For this review, take the finished solid that the model builds, in its own axes (mm). Face numbers are marked on the shaded views. A direction names the side the tool comes from. Coordinates: 2 decimals unless noted, no trailing zeros. Loops run counter-clockwise (first coordinate to the right, second up) from the corner with the lowest first, then second, coordinate; pieces in that order, holes last. Notation, with made-up numbers: M 43,-16.75 L 63,-16.75 A25 ccw 63,6.25 Z; hole C 54,1.25 d2. An arc over 180 degrees is marked long. Answer as a JSON object with one key per item and string values. Group by question number.
Item 1: Mouldability with a two-part tool opening along X and no side actions: class the marked faces 4, 5 and 6 as +X half, -X half, draft (parallel to the pull), parting line (faces both ways), or undercut.
Item 2: Add section A-A (y = 80). State the section outline as (x, z) points.
Item 3: Add section B-B (z = -171). State the section outline as (x, y) points, then the cut area to 3 significant figures.
Item 4: Add section C-C (x = 119). State the section outline as (y, z) points.
Item 5: Wall thickness on L1, parallel to Z at x = 210.5, y = 64.5; L2, parallel to X at y = 118.5, z = -390; L3, parallel to X at y = 9, z = -358: over which ranges is each line inside the solid? List them lowest first. Write a range as from..to.
Item 6: Insertion check: pin 1 (1 mm diameter, centred on y = 116, z = -232, fed in from +X); pin 2 (5 mm diameter, centred on x = 156, z = -265, fed in from +Y); pin 3 (8 mm diameter, centred on y = 132, z = -338.5, fed in from -X). Each pin has a flat end and moves straight along its axis. Give the tip position at first contact, or say it passes through.
Item 7: Tool access review of the marked faces 1, 2 and 3: name each direction out of +Z, -Z, +X, -X, +Y, -Y from which nothing blocks a thin tool from reaching the whole face with its end or side.
Autodesk Inventor part; units mm, degrees
ref_plane "YZ Plane" through (0, 0, 0) normal (1, 0, 0) x (0, 1, 0)
ref_plane "XZ Plane" through (0, 0, 0) normal (0, 1, 0) x (-1, 0, 0)
ref_plane "XY Plane" through (0, 0, 0) normal (0, 0, 1) x (1, 0, 0)
sketch "Sketch5" plane through (0, 0, 0) normal (0, 0, 1) x (1, 0, 0)
  line L0 (0, 0) -> (370, 0)
  line L1 (370, 0) -> (370, 150)
  line L2 (370, 150) -> (0, 150)
  line L3 (0, 150) -> (0, 0)
  dimension "d15" = 370
  dimension "d16" = 150
extrude "Extrusion5" add sketch "Sketch5" along normal blind 18
sketch "Sketch6" plane through (0, 0, 0) normal (0, 0, -1) x (-1, 0, 0)
  line L0 (-362.3, 140) -> (-344.3, 140)
  line L1 (-344.3, 140) -> (-344.3, 5)
  line L2 (-344.3, 5) -> (-362.3, 5)
  line L3 (-362.3, 5) -> (-362.3, 140)
  line L4 (-370, 0) -> (-370, 150)
  line L5 (0, 0) -> (-370, 0)
  line L6 (-25.7, 140) -> (-7.7, 140)
  line L7 (-7.7, 140) -> (-7.7, 5)
  line L8 (-7.7, 5) -> (-25.7, 5)
  line L9 (-25.7, 5) -> (-25.7, 140)
  line L10 (0, 150) -> (0, 0)
  dimension "d19" = 18
  dimension "d20" = 135
  dimension "d21" = 7.7
  dimension "d22" = 5
  dimension "d23" = 18
  dimension "d24" = 7.7
  dimension "d25" = 5
extrude "Extrusion6" add sketch "Sketch6" along normal blind 550
sketch "Sketch7" plane through (0, 0, -550) normal (0, 0, -1) x (-1, 0, 0)
  line L0 (-344.3, 140) -> (-344.3, 5)
  line L1 (-25.7, 5) -> (-25.7, 140)
  line L2 (-344.3, 140) -> (-25.7, 140)
  line L3 (-25.7, 140) -> (-25.7, 5)
  line L4 (-25.7, 5) -> (-344.3, 5)
  line L5 (-344.3, 5) -> (-344.3, 140)
  point P0 (0, 0)
extrude "Extrusion7" add sketch "Sketch7" against normal blind 18
sketch "Sketch8" plane through (7.7, 5, -550) normal (0, -1, 0) x (1, 0, 0)
  line L0 (354.6, 550) -> (336.6, 550)
  line L1 (354.6, 550) -> (354.6, 0)
  line L2 (0, 0) -> (354.6, 0)
  line L3 (0, 550) -> (0, 0)
  line L4 (18, 550) -> (0, 550)
  line L5 (18, 550) -> (18, 18)
  line L6 (336.6, 18) -> (18, 18)
  line L7 (336.6, 550) -> (336.6, 18)
  line L8 (362.3, 550) -> (-7.7, 550)
extrude "Extrusion8" add sketch "Sketch8" against normal blind 9 contours L7 L6 L5 L8
equation "\"d16\" = Cajon02Altura"
equation "\"d24\" = d21"
equation "\"d25\" = d22"
properties part number "FrenteGrande" material "Wood (Birch)"
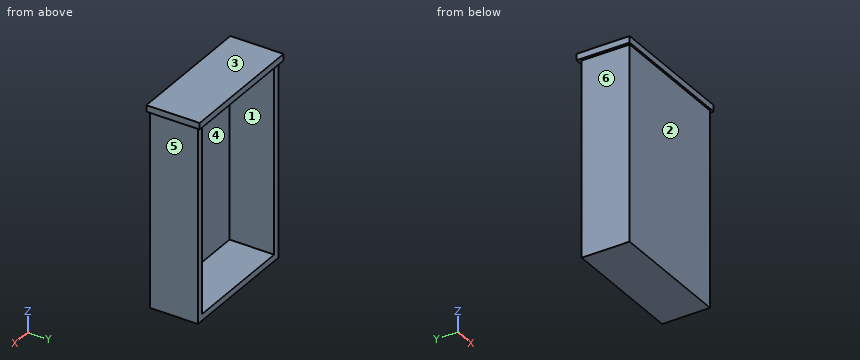
From the geometry:
{
 "1": {"face 4": "undercut", "face 5": "+X half", "face 6": "-X half"},
 "2": {"outline": "M 0,0 L 7.7,0 L 7.7,-550 L 362.3,-550 L 362.3,0 L 370,0 L 370,18 L 0,18 Z; hole M 25.7,-532 L 344.3,-532 L 344.3,0 L 25.7,0 Z"},
 "3": {"outline": "M 7.7,5 L 362.3,5 L 362.3,140 L 344.3,140 L 344.3,14 L 25.7,14 L 25.7,140 L 7.7,140 Z", "area": "7,730 mm²"},
 "4": {"outline": "M 0,0 L 5,0 L 5,-550 L 140,-550 L 140,-532 L 14,-532 L 14,0 L 150,0 L 150,18 L 0,18 Z"},
 "5": {"L1": "z = -550..-532, 0..18", "L2": "x = 7.7..25.7, 344.3..362.3", "L3": "x = 7.7..362.3"},
 "6": {"pin 1": "stops at x = 362.3", "pin 2": "stops at y = 14", "pin 3": "stops at x = 7.7"},
 "7": {"face 1": "+Y", "face 2": "-Z, +X, -X, -Y", "face 3": "+Z, +X, -X, +Y, -Y"}
}
